Geometry: see drawing. Coordinates: mm, zero at the bounding-box minimum. Round coordinates to 2 decimals unless told otherwise and drop trailing zeros. Loops run counter-clockwise (first coordinate to the right, second up) from the corner with the lowest first, then second, coordinate; pieces in that order, holes last. Notation, with made-up numbers: (55, -12) - (65, -12) arc R26 ccw to (65, 3) - close; hole circle Ø8 at (-4, 66.25). An arc over 180 degrees is marked (long way). Use CSV: the item, a comma, the result in double quotes.
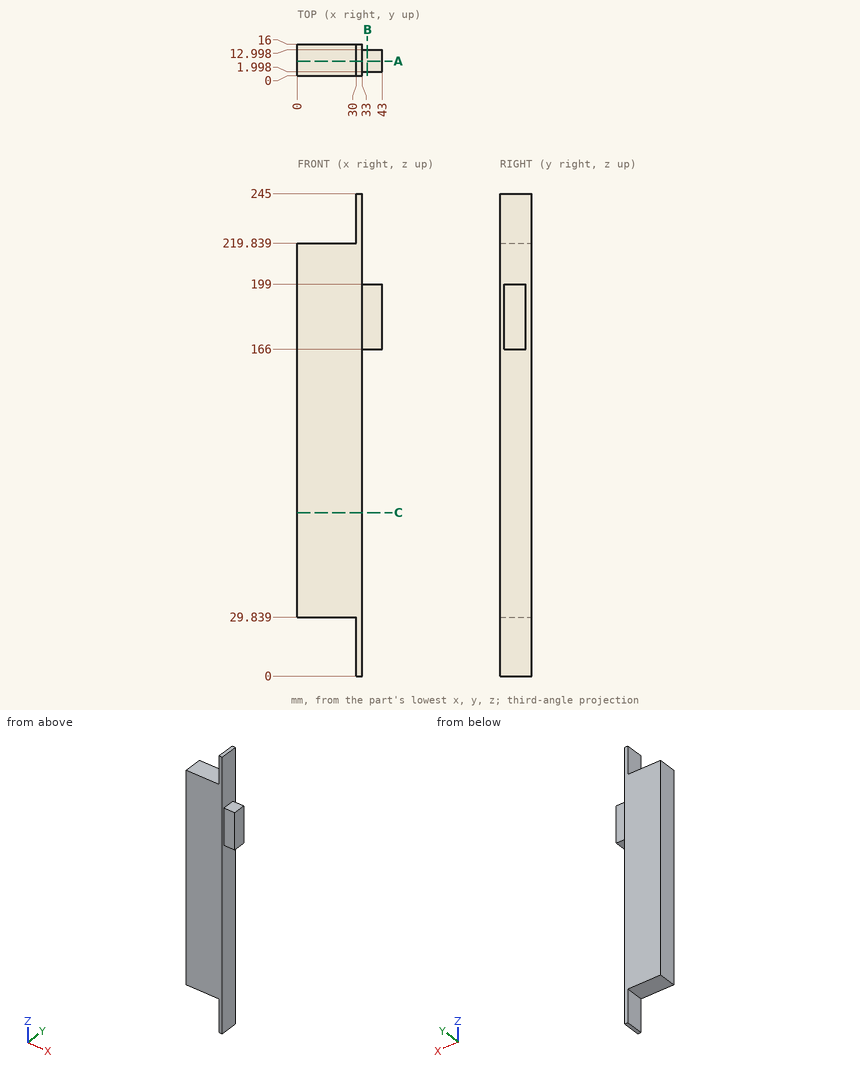
Item 1: Section B-B on x = 35.5. Return the cut outline in (y, z).
Final values:
outline,"(2, 166) - (13, 166) - (13, 199) - (2, 199) - close"
Item 2: Material intervals for line 1 (X direction, y = 1.5, z = 49); line 2 (Z direction, x = 10.5, y = 1.5); line 3 (X direction, y = 15, z = 230), sorted ascending.
Final values:
line 1,"x = 0 to 33"
line 2,"z = 29.84 to 219.84"
line 3,"x = 30 to 33"
Item 3: Section A-A on y = 7.25. Return the cut outline in (x, z), plus the area to 4 significant figures.
Final values:
outline,"(0, 29.84) - (30, 29.84) - (30, 0) - (33, 0) - (33, 166) - (43, 166) - (43, 199) - (33, 199) - (33, 245) - (30, 245) - (30, 219.84) - (0, 219.84) - close"
area,"6,765 mm²"
Item 4: Section C-C on z = 83. Return the cut outline in (x, y).
Final values:
outline,"(0, 0) - (33, 0) - (33, 16) - (0, 16) - close"
Item 5: Pin query (flat end, axial travel): P1, Ø3, axis at x = 37.5, y = 8, coming from the -Z side; P2, Ø1, axis at x = 9.5, y = 6.5, coming from the +Z side; P3, Ø8, axis at y = 10.5, z = 237.5, coming from the -X side. Return the tip coordinate at first contact, or that it passes through.
Final values:
P1,"stops at z = 166"
P2,"stops at z = 219.84"
P3,"stops at x = 30"
